Verification items for the finished model (mm, model axes). Face numbers are marked on the shaded views. A direction names the side the tool comes from. Coordinates: 2 decimals unless noted, no trailing zeros. Loops run counter-clockwise (first coordinate to the right, second up) from the corner with the lowest first, then second, coordinate; pieces in that order, holes last. Notation, with made-up numbers: (-2.75, 74.5) -> (28.25, 74.5) arc R24 ccw to (28.25, 98.5) -> close; hole circle Ø5 at (-23, 87.25). An arc over 180 degrees is marked (long way). Write item = value, one per line.
```python
from build123d import *

# Parameters (mm, degrees)
F0_R     = 32.5
F1_DEPTH = 12
F2_R     = 17.5
F3_DEPTH = 10
F4_R     = 9
F5_DEPTH = 2000
F7_D     = 6
F7_DEPTH = 32.501
F9_D     = 3


with BuildPart() as f1:
    # F0 (on Top) → F1 (new body)
    with BuildSketch(Plane.XY):
        Circle(F0_R)
    extrude(amount=F1_DEPTH)

    # F2 (on face) → F3 (cut)
    with BuildSketch(Plane.XY.offset(12)):
        Circle(F2_R)
    extrude(amount=-F3_DEPTH, mode=Mode.SUBTRACT)

    # F4 (on face) → F5 (cut)
    with BuildSketch(Plane.XY.offset(2)):
        Circle(F4_R)
    extrude(amount=-F5_DEPTH, mode=Mode.SUBTRACT)

    # F7 (through all, one way)
    with BuildSketch(Plane(origin=(0, 0, 0), x_dir=(1, 0, 0), z_dir=(0, 1, 0))):
        with Locations((0, -6)):
            Circle(F7_D / 2)
    extrude(amount=-F7_DEPTH, mode=Mode.SUBTRACT)

    # F9 (through all)
    with Locations(Plane.XY.offset(12)):
        with Locations((0, -27.5)):
            Hole(F9_D / 2)


solid = f1.part
```
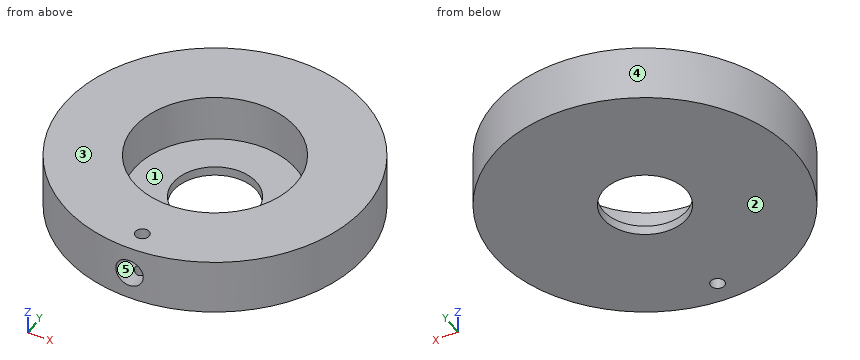
1) Material ranges on line 1 (Y direction, x = 0, z = 1.85); line 2 (Y direction, x = 0, z = 2.75); line 3 (Y direction, x = -9, z = 8), recorded low to high.
Ans:
line_1 = -32.5 to -29, -26 to -9, 9 to 32.5
line_2 = -32.5 to -29, -26 to -17.5, 17.5 to 32.5
line_3 = -31.23 to -15.01, 15.01 to 31.23
2) Tool access check on the marked faces 1 and 2. Record the directions out of +Z, -Z, +X, -X, +Y, -Y that give a thin tool (end or side, any length) a straight path to the whole face; none if there is none.
Ans:
face_1 = +Z
face_2 = -Z, +X, -X, +Y, -Y
3) Sectioned sample at A-A, the plane y = 0. Record the cut outline in (x, z), plus the area to 3 significant figures.
Ans:
outline = (-32.5, 0) -> (-9, 0) -> (-9, 2) -> (-17.5, 2) -> (-17.5, 12) -> (-32.5, 12) -> close; (9, 0) -> (32.5, 0) -> (32.5, 12) -> (17.5, 12) -> (17.5, 2) -> (9, 2) -> close
area = 394 mm2
4) Release check for a two-part mould opening along X. For the marked faces 3, 4 and 5 record: pulls with the +X half, pulls with the -X half, needs draft (parallel to the pull), parting line crosses it, or undercut.
Ans:
face_3 = needs draft
face_4 = parting line crosses it
face_5 = undercut
5) Sectioned sample at C-C, the plane x = 8. Record the cut outline in (y, z), plus the area to 3 significant figures.
Ans:
outline = (-31.5, 0) -> (-4.12, 0) -> (-4.12, 2) -> (-15.56, 2) -> (-15.56, 12) -> (-31.5, 12) -> close; (4.12, 0) -> (31.5, 0) -> (31.5, 12) -> (15.56, 12) -> (15.56, 2) -> (4.12, 2) -> close
area = 428 mm2
6) Depth check by flat-ended pin: pin 1 Ø17.5 at (x, y) = (-7, -5) entering from +Z; pin 2 Ø1 at (x, z) = (-26, 5.5) entering from -Y; pin 3 Ø6 at (x, z) = (-11, 7) entering from +Y. Enter the tip coordinate at first touch or a pass-through.
Ans:
pin_1 = 2
pin_2 = -20.15
pin_3 = 31.5
7) Sectioned sample at B-B, the plane x = 0. Record the cut outline in (y, z).
Ans:
outline = (-32.5, 0) -> (-29, 0) -> (-29, 3) -> (-32.5, 3) -> close; (-32.5, 9) -> (-29, 9) -> (-29, 12) -> (-32.5, 12) -> close; (-26, 0) -> (-9, 0) -> (-9, 2) -> (-17.5, 2) -> (-17.5, 3) -> (-26, 3) -> close; (-26, 9) -> (-17.5, 9) -> (-17.5, 12) -> (-26, 12) -> close; (9, 0) -> (32.5, 0) -> (32.5, 12) -> (17.5, 12) -> (17.5, 2) -> (9, 2) -> close
8) Sectioned sample at D-D, the plane x = 28. Record the cut outline in (y, z), plus the area to 3 significant figures.
Ans:
outline = (-16.5, 0) -> (16.5, 0) -> (16.5, 12) -> (-16.5, 12) -> close
area = 396 mm2
